Verification items for this drawing (mm, ordinates from the low corner). Give positions to 0.01 mm unless a question says otherwise; leave off trailing zeros. Loops run counter-clockwise (first coordinate to the right, second up) from the corner with the lowest first, then second, coordinate; pieces in that order, holes last. Notation, with made-up numbers: (22.25, -36.5) -> (75.25, -36.5) arc R16 ccw to (75.25, -28.5) -> close; hole circle Ø2 at (84, 80.25). An arc over 180 degrees is marked (long way). Answer as a JSON object with one key per item and string values.
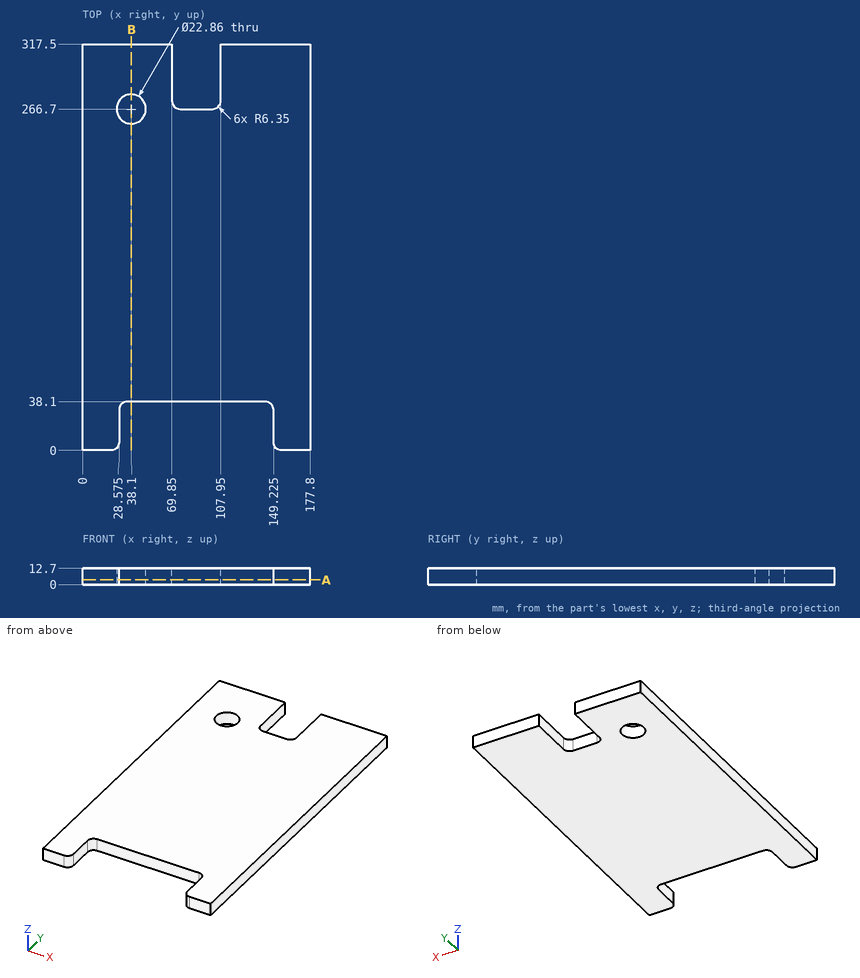
1) Section check B-B on x = 38.1. Record the cut outline in (y, z), plus the area to 3 significant figures.
Geometry check:
{"outline": "(38.1, 0) -> (255.27, 0) -> (255.27, 12.7) -> (38.1, 12.7) -> close; (278.13, 0) -> (317.5, 0) -> (317.5, 12.7) -> (278.13, 12.7) -> close", "area": "3,260 mm2"}
2) Material ranges on line 1 along Y through (x, z) = (38.1, 8.75); line 2 along X through (y, z) = (19, 5.5) (3 decimals); line 3 along Y through (x, z) = (66, 2), recorded low to high. Write a range as from..to.
Geometry check:
{"line 1": "y = 38.1..255.27, 278.13..317.5", "line 2": "x = 0..28.575, 149.225..177.8", "line 3": "y = 38.1..317.5"}
3) Section check A-A on z = 3.75. Record the cut outline in (x, y) (3 decimals), plus the area to 3 significant figures.
Geometry check:
{"outline": "(0, 0) -> (22.225, 0) arc R6.35 ccw to (28.575, 6.35) -> (28.575, 31.75) arc R6.35 cw to (34.925, 38.1) -> (142.875, 38.1) arc R6.35 cw to (149.225, 31.75) -> (149.225, 6.35) arc R6.35 ccw to (155.575, 0) -> (177.8, 0) -> (177.8, 317.5) -> (107.95, 317.5) -> (107.95, 273.05) arc R6.35 cw to (101.6, 266.7) -> (76.2, 266.7) arc R6.35 cw to (69.85, 273.05) -> (69.85, 317.5) -> (0, 317.5) -> close; hole circle Ø22.86 at (38.1, 266.7)", "area": "49,500 mm2"}
4) Depth check by flat-ended pin: P1, Ø6, axis at x = 83.5, z = 3, coming from the -Y side. Enter the tip coordinate at first touch or a pass-through.
Geometry check:
{"P1": "stops at y = 38.1"}
